```python
from build123d import *

# Parameters (mm, degrees)
F0_W     = 10.45
F0_H     = 24.72
F1_DEPTH = 8.22
F2_R     = 0.845507
F3_DEPTH = 1.37


with BuildPart() as f1:
    # F0 (on Top) → F1 (new body)
    with BuildSketch(Plane.XY):
        with Locations((-27.746155, -7.76654)):
            Rectangle(F0_W, F0_H)
    extrude(amount=-F1_DEPTH)

    # F2 (on Top) → F3 (join)
    with BuildSketch(Plane.XY):
        with Locations((-24.125788, -19.778986)):
            Circle(F2_R)
    extrude(amount=-F3_DEPTH)


solid = f1.part
```
Check sheet for the modelled part. Datum: model origin and axes. Units: mm. Round coordinates to 2 decimals unless told otherwise and drop trailing zeros. Write each loop counter-clockwise with the first axis right and the second up, starting at its lowest first coordinate (ties: lowest second). Pieces come first, ordered by that corner, then holes. Notation, with made-up numbers: (74, 58) -> (97, 58) arc R17 cw to (97, 88) -> close; hole circle Ø9 at (4.5, 31.5). An arc over 180 degrees is marked (long way). Put each result on its own line as item: value.
(1) Sectioned sample at C-C (z = -3.25). Enter the section's corners in (x, y).
Values found:
outline: (-32.97, -20.13) -> (-22.52, -20.13) -> (-22.52, 4.59) -> (-32.97, 4.59) -> close
(2) Go/stop test with a flat-tipped pin: pin 1 Ø2.5 at (x, z) = (-30, -2) entering from -Y. Record where the tip stops, or that it passes through.
Values found:
pin 1: stops at y = -20.13
(3) Sectioned sample at D-D (x = -24). Enter the section's corners in (y, z).
Values found:
outline: (-20.62, -1.37) -> (-20.13, -1.37) -> (-20.13, -8.22) -> (4.59, -8.22) -> (4.59, 0) -> (-20.62, 0) -> close
(4) Material ranges on line 1 (Y direction, x = -27.25, z = -1.75), recorded low to high.
Values found:
line 1: y = -20.13 to 4.59
(5) Sectioned sample at B-B (x = -32). Enter the section's corners in (y, z).
Values found:
outline: (-20.13, -8.22) -> (4.59, -8.22) -> (4.59, 0) -> (-20.13, 0) -> close
(6) Sectioned sample at A-A (z = -0.5). Enter the section's corners in (x, y).
Values found:
outline: (-32.97, -20.13) -> (-24.9, -20.13) arc R0.85 ccw to (-23.36, -20.13) -> (-22.52, -20.13) -> (-22.52, 4.59) -> (-32.97, 4.59) -> close
